Work out the finished part from the listing and answer in its coordinate system (mm). A direction names the side the tool comes from. Coordinates: 2 decimals unless noted, no trailing zeros. Write each loop counter-clockwise with the first axis right and the second up, starting at its lowest first coordinate (ties: lowest second). Pieces come first, ordered by that corner, then holes. Notation, with made-up numbers: (58.5, -6) - (97.5, -6) arc R21 ccw to (97.5, 13) - close; hole circle Ø1 at (73, -34.75). An arc over 180 degrees is marked (long way). Use a Markdown table: item, result. Add a question column.
(1) A tool of negligible diameter and unlimited length cuts with its end or side. For faces 4 (the face through (0.567, 1.088, 0.616)), 5 (the face through (6, 0, 0)), from which of +Z, -Z, +X, -X, +Y, -Y can it reach the whole face along a straight path? Write none if from no direction.
(2) Given pin 1 Ø1 at (x, y) = (1, -3) entering from +Z; pin 2 Ø1 at (x, y) = (2.5, -1) entering from -Z; pin 3 Ø0.9 at (x, y) = (1, 0) entering from +Z, each flat-ended and moving along its own axis, determine where each tip first touches the part or whether it passes through.
(3) The part is cut by section B-B, the plane y = 0. Give the vertices of the cut face in (x, z).
(4) The part is cut by section C-C, the plane x = 4.4. Give the vertices of the cut face in (y, z).
(5) For a pull along Z with two mould halves and no side action, classify faces 1 (the face through (0.6, 0, 1.25)), 2 (the face through (0, 2, 0)), 3 (the face through (4, 0, -2)) as released by +Z, released by -Z, zero draft, split by the parting line, or undercut.
(6) The part is cut by section A-A, the plane x = 0.6. Give the vertices of the cut face in (y, z), then the cut area to 3 significant figures.
(7) Find the intervals of material crossed by line 1 (Y direction, x = 0.4, z = 1); line 2 (X direction, y = -2.25, z = -1); line 3 (X direction, y = 3, z = -1.5), in increasing order. Write a range as from..to.
Autodesk Inventor part; units mm, degrees
ref_plane "YZ Plane" through (0, 0, 0) normal (1, 0, 0) x (0, 1, 0)
ref_plane "XZ Plane" through (0, 0, 0) normal (0, 1, 0) x (-1, 0, 0)
ref_plane "XY Plane" through (0, 0, 0) normal (0, 0, 1) x (1, 0, 0)
sketch "__1" plane through (0, 0, 0) normal (0, 0, 1) x (1, 0, 0)
  line L0 (56, 0) -> (-56, 0)
  line L1 (0, 0) -> (0, 4)
  line L2 (0, 4) -> (2, 2)
  line L3 (2, 2) -> (5.5705, 2)
  line L4 (5.5705, 2) -> (6, 1.5705)
  line L5 (6, 1.5705) -> (6, 0)
  line L6 (6, 0) -> (0, 0)
revolve "Revolution1" add sketch "__1" angle 360 about axis through (56, 0, 0) along (1, 0, 0)
thread "Thread1"
sketch "__2" plane through (0, 0, 0) normal (1, 0, 0) x (0, 0, -1)
  line L0 (-1.25, -0.7217) -> (0, -1.4434)
  line L1 (0, -1.4434) -> (1.25, -0.7217)
  line L2 (1.25, -0.7217) -> (1.25, 0.7217)
  line L3 (1.25, 0.7217) -> (0, 1.4434)
  line L4 (0, 1.4434) -> (-1.25, 0.7217)
  line L5 (-1.25, 0.7217) -> (-1.25, -0.7217)
extrude "Extrusion1" cut sketch "__2" along normal blind 1.15
fillet "Fillet1" radius 0.05 1 edges at (0, -4, 0)
properties part number "FBB4-6" material "Steel"
Model answer:
| question | item | result |
|---|---|---|
| 1 | face 4 | -X |
| 1 | face 5 | +Z, -Z, +X, +Y, -Y |
| 2 | pin 1 | z = 2.07 |
| 2 | pin 2 | z = -1.94 |
| 2 | pin 3 | z = 3.45 |
| 3 | outline | (0, -3.88) arc R0.05 ccw to (0.09, -3.91) - (2, -2) - (5.57, -2) - (6, -1.57) - (6, 1.57) - (5.57, 2) - (2, 2) - (0.09, 3.91) arc R0.05 ccw to (0, 3.88) - (0, 1.25) - (1.15, 1.25) - (1.15, -1.25) - (0, -1.25) - close |
| 4 | outline | circle Ø4 at (0, 0) |
| 5 | face 1 | undercut |
| 5 | face 2 | zero draft |
| 5 | face 3 | split by the parting line |
| 6 | outline | circle Ø6.8 at (0, 0); hole (-1.44, 0) - (-0.72, -1.25) - (0.72, -1.25) - (1.44, 0) - (0.72, 1.25) - (-0.72, 1.25) - close |
| 6 | area | 30.9 mm^2 |
| 7 | line 1 | -3.46..-0.87, 0.87..3.46 |
| 7 | line 2 | 0..1.54 |
| 7 | line 3 | 0..0.65 |
